```python
from build123d import *

# Parameters (mm, degrees)
SKETCH1_W           = 70
SKETCH1_H           = 35
BOSS_EXTRUDE1_DEPTH = 37
SHELL1_T            = -2
CUT_EXTRUDE1_DEPTH  = 2
SKETCH3_W           = 60
SKETCH3_H           = 30
CUT_EXTRUDE3_DEPTH  = 2
SKETCH4_W           = 60
SKETCH4_H           = 3
CUT_EXTRUDE4_DEPTH  = 2
SKETCH5_R           = 2.5
CUT_EXTRUDE5_DEPTH  = 2
CUT_EXTRUDE6_START  = -2
SKETCH6_R           = 2.5
CUT_EXTRUDE6_DEPTH  = 2


with BuildPart() as part:
    # Sketch1 → Boss-Extrude1 (new body)
    with BuildSketch(Plane(origin=(0, 0, 0), x_dir=(1, 0, 0), z_dir=(0, 1, 0))):
        with Locations((-44.968255968, 17.192111045)):
            Rectangle(SKETCH1_W, SKETCH1_H)
    extrude(amount=BOSS_EXTRUDE1_DEPTH)

    # Shell1
    shell1_openings = [part.faces().sort_by_distance(p)[0] for p in [
        (-44.968255968, 0, -17.192111045),
    ]]
    offset(amount=SHELL1_T, openings=shell1_openings, kind=Kind.INTERSECTION)

    # Sketch2 → Cut-Extrude1 (cut)
    with BuildSketch(Plane.XY.offset(0.307888955)):
        with BuildLine():
            Line((-45.968255968, 0), (-44.968255968, 0))
            Line((-44.968255968, 0), (-43.968255968, 0))
            ThreePointArc((-43.968255968, 0), (-44.968255968, 1), (-45.968255968, 0))
        make_face()
    extrude(amount=-CUT_EXTRUDE1_DEPTH, mode=Mode.SUBTRACT)

    # Sketch3 → Cut-Extrude3 (cut)
    with BuildSketch(Plane(origin=(0, 0, -34.692111045), x_dir=(-1, 0, 0), z_dir=(0, 0, -1))):
        with Locations((44.968255968, 15)):
            Rectangle(SKETCH3_W, SKETCH3_H)
    extrude(amount=-CUT_EXTRUDE3_DEPTH, mode=Mode.SUBTRACT)

    # Sketch4 → Cut-Extrude4 (cut)
    with BuildSketch(Plane.XY.offset(0.307888955)):
        with Locations((-44.968255968, 14.5)):
            Rectangle(SKETCH4_W, SKETCH4_H)
        with Locations((-44.968255968, 22.5)):
            Rectangle(SKETCH4_W, SKETCH4_H)
        with Locations((-44.968255968, 30.5)):
            Rectangle(SKETCH4_W, SKETCH4_H)
        with Locations((-44.968255968, 6.5)):
            Rectangle(SKETCH4_W, SKETCH4_H)
    extrude(amount=-CUT_EXTRUDE4_DEPTH, mode=Mode.SUBTRACT)

    # Sketch5 → Cut-Extrude5 (cut)
    with BuildSketch(Plane.ZY.offset(79.968255968)):
        with Locations((-26.149373003, 28.09173468)):
            Circle(SKETCH5_R)
        with Locations((-26.149373003, 19.50769197)):
            Circle(SKETCH5_R)
        with Locations((-26.149373003, 10.401142313)):
            Circle(SKETCH5_R)
        with Locations((-16.445672549, 10.401142313)):
            Circle(SKETCH5_R)
        with Locations((-16.445672549, 19.50769197)):
            Circle(SKETCH5_R)
        with Locations((-16.445672549, 28.09173468)):
            Circle(SKETCH5_R)
        with Locations((-7.339122891, 28.09173468)):
            Circle(SKETCH5_R)
        with Locations((-7.339122891, 19.50769197)):
            Circle(SKETCH5_R)
        with Locations((-7.339122891, 10.401142313)):
            Circle(SKETCH5_R)
    extrude(amount=-CUT_EXTRUDE5_DEPTH, mode=Mode.SUBTRACT)

    # Sketch6 → Cut-Extrude6 (cut)
    with BuildSketch(Plane(origin=(-9.968255968, 0, 0), x_dir=(0, 0, -1), z_dir=(1, 0, 0)).offset(CUT_EXTRUDE6_START)):
        with Locations((7.264479042, 28.09173468)):
            Circle(SKETCH6_R)
        with Locations((7.264479042, 19.50769197)):
            Circle(SKETCH6_R)
        with Locations(Location((7.339122891, 10.401142313, 0), (0, 0, 180))):
            Circle(SKETCH6_R)
        with Locations(Location((16.445672549, 10.401142313, 0), (0, 0, 180))):
            Circle(SKETCH6_R)
        with Locations(Location((16.445672549, 19.50769197, 0), (0, 0, 180))):
            Circle(SKETCH6_R)
        with Locations(Location((26.149373003, 19.50769197, 0), (0, 0, 180))):
            Circle(SKETCH6_R)
        with Locations(Location((16.445672549, 28.09173468, 0), (0, 0, 180))):
            Circle(SKETCH6_R)
        with Locations(Location((26.149373003, 28.09173468, 0), (0, 0, 180))):
            Circle(SKETCH6_R)
        with Locations(Location((26.149373003, 10.401142313, 0), (0, 0, 180))):
            Circle(SKETCH6_R)
    extrude(amount=CUT_EXTRUDE6_DEPTH, mode=Mode.SUBTRACT)


solid = part.part
```
Build history of the part. All positions in model axes, mm. A direction names the side the tool comes from. Coordinates: 2 decimals unless noted, no trailing zeros. Order: outer loops, then holes, each group sorted by start corner. A loop starts at its lowest first (then second) coordinate and runs counter-clockwise, first axis right, second up. Notation, with made-up numbers: M 40,-10 L 93,-10 A23 cw 93,6 Z; hole C -16.75,3.25 d1. An arc over 180 degrees is marked long. One line per question, with ' | ' between items. Start each with the question number.
1. Tool access for faces 1 (the face through (-78.98, 25.87, -6.19)), 2 (the face through (-10.98, 20.26, -9.65)), 3 (the face through (-11.968, 17, -14)), 4 (the face through (-74.968, 22, -1)): list every direction of +Z, -Z, +X, -X, +Y, -Y with a clear straight run to the whole face (end or side of a thin tool).
2. Flat gauge pins, fed straight in: P1, Ø3, axis at y = 28.09, z = -16.45, coming from the +X side; P2, Ø5, axis at x = -29.5, y = 24.5, coming from the -Z side; P3, Ø0.6, axis at x = -52.5, z = -33.5, coming from the -Y side; P4, Ø4, axis at x = -33.5, z = -14.5, coming from the -Y side. Where does each tip first touch, or does it go through?
3. Cut at B-B (y = 15). Write the cut outline in (x, z).
4. Mould opens along X. For faces 5 (the face through (-9.968, 22.4, -16.9)), 6 (the face through (-10.98, 30.31, -15.29)), 7 (the face through (-45, 29, -1)) say: +X half, -X half, draft (parallel to the pull), parting line (faces both ways), or undercut.
5. Cut at D-D (z = -11.5). Write the cut outline in (x, y), plus the area to 3 significant figures.
6. Cut at A-A (x = -50.5). Write the cut outline in (y, z), plus the area to 3 significant figures.
7. Wall check: line 1 along X through (y, z) = (16, -8); line 2 along Z through (x, y) = (-14, 23); line 3 along Z through (x, y) = (-36, 19). Give the ranges that are in metal, low to high. Write a range as [from, to].
8. Cut at C-C (z = -25). Count the separate pieces of the cut face and the enclosed holes in it, plus the area to 3 significant figures.
The answers:
1) face 1: -X | face 2: +X | face 3: -Y | face 4: +Z, -Z
2) P1: passes through | P2: stops at z = -1.69 | P3: stops at y = 30 | P4: stops at y = 35
3) outline: M -79.97,-34.69 L -74.97,-34.69 L -74.97,-32.69 L -77.97,-32.69 L -77.97,-1.69 L -74.97,-1.69 L -74.97,0.31 L -79.97,0.31 Z; M -14.97,-34.69 L -9.97,-34.69 L -9.97,0.31 L -14.97,0.31 L -14.97,-1.69 L -11.97,-1.69 L -11.97,-32.69 L -14.97,-32.69 Z
4) face 5: +X half | face 6: draft | face 7: undercut
5) outline: M -79.97,0 L -77.97,0 L -77.97,35 L -11.97,35 L -11.97,0 L -9.97,0 L -9.97,37 L -79.97,37 Z | area: 280 mm2
6) outline: M 0,-1.69 L 5,-1.69 L 5,0.31 L 0,0.31 Z; M 8,-1.69 L 13,-1.69 L 13,0.31 L 8,0.31 Z; M 16,-1.69 L 21,-1.69 L 21,0.31 L 16,0.31 Z; M 24,-1.69 L 29,-1.69 L 29,0.31 L 24,0.31 Z; M 30,-34.69 L 37,-34.69 L 37,0.31 L 32,0.31 L 32,-1.69 L 35,-1.69 L 35,-32.69 L 30,-32.69 Z | area: 126 mm2
7) line 1: x = [-79.97, -77.97], [-11.97, -9.97] | line 2: z = [-34.69, -32.69], [-1.69, 0.31] | line 3: z = [-1.69, 0.31]
8) separate pieces: 7 | enclosed holes: 0 | area: 227 mm2
